```python
from build123d import *

# Parameters (mm, degrees)
SKETCH1_R          = 5.25
SKETCH1_R_2        = 10
SKETCH1_R_3        = 6.25
SKETCH1_R_4        = 4.25
BASE_FLANGE1_DEPTH = 4
FILLET1_R          = 10


# Sheet-metal steps are written as plain solids
with BuildPart() as part:
    # Sketch1 → Base-Flange1 (new body)
    with BuildSketch(Plane(origin=(0, 0, 0), x_dir=(1, 0, 0), z_dir=(0, 1, 0))):
        Polygon((70, -42.5), (-70, -42.5), (-70, 42.5), (-70, 72.5), (230, 72.5), (230, 42.5), (70, 42.5), align=None)
        with Locations(Location((-55, 57.5, 0), (0, 0, 270))):
            Circle(SKETCH1_R, mode=Mode.SUBTRACT)
        with Locations(Location((215, 57.5, 0), (0, 0, 270))):
            Circle(SKETCH1_R, mode=Mode.SUBTRACT)
        with Locations(Location((0, -17.5, 0), (0, 0, 270))):
            Circle(SKETCH1_R_2, mode=Mode.SUBTRACT)
        with Locations(Location((-45, -17.5, 0), (0, 0, 270))):
            Circle(SKETCH1_R_3, mode=Mode.SUBTRACT)
        with Locations(Location((45, -17.5, 0), (0, 0, 270))):
            Circle(SKETCH1_R_3, mode=Mode.SUBTRACT)
        with Locations(Location((-45, 12.5, 0), (0, 0, 270))):
            Circle(SKETCH1_R_4, mode=Mode.SUBTRACT)
        with Locations(Location((45, 12.5, 0), (0, 0, 270))):
            Circle(SKETCH1_R_4, mode=Mode.SUBTRACT)
    extrude(amount=-BASE_FLANGE1_DEPTH)

    # Fillet1
    fillet1_edges = [part.edges().sort_by_distance(p)[0] for p in [
        (-70, -2, -72.5),
        (230, -2, -72.5),
        (230, -2, -42.5),
        (70, -2, -42.5),
        (70, -2, 42.5),
        (-70, -2, 42.5),
    ]]
    fillet(fillet1_edges, radius=FILLET1_R)


solid = part.part
```
Source: CAD feature listing. Evaluate the final solid. Frame: model axes, mm. Give positions to 0.01 mm unless a question says otherwise; leave off trailing zeros. Write each loop counter-clockwise with the first axis right and the second up, starting at its lowest first coordinate (ties: lowest second). Pieces come first, ordered by that corner, then holes.
1. Section query B-B (z = 17.5). Return the cut outline in (x, y), then the cut area to 3 significant figures.
2. Section query D-D (z = -57.5). Return the cut outline in (x, y), then the cut area to 3 significant figures.
3. First-contact query: pin 1 (7 mm diameter, centred on x = 45, z = -12.5, fed in from -Y); pin 2 (2 mm diameter, centred on y = -1.5, z = -10, fed in from +X). Flat tips, straight axial feed; report the tip coordinate or a pass-through.
4. Pull-direction query (Z, two-part tool) for faces 1 (the face through (66.99, -2.03, 39.65)), 2 (the face through (-67.15, -2.03, -69.49)), 3 (the face through (51.2, -2, 16.7)); classes: +Z half, -Z half, draft (parallel to the pull), parting line (faces both ways), or undercut.
5. Section query C-C (x = 45). Return the cut outline in (y, z), then the cut area to 3 significant figures.
6. Material intervals for line 1 along X through (y, z) = (-0.95, 17.5); line 2 along X through (y, z) = (-2.05, -57.5); line 3 along X through (y, z) = (-2.8, 15.5), sorted ascending.
7. Section query A-A (x = 0). Return the cut outline in (y, z), then the cut area to 3 significant figures.
Output values:
1. outline: (-70, -4) - (-51.25, -4) - (-51.25, 0) - (-70, 0) - close; (-38.75, -4) - (-10, -4) - (-10, 0) - (-38.75, 0) - close; (10, -4) - (38.75, -4) - (38.75, 0) - (10, 0) - close; (51.25, -4) - (70, -4) - (70, 0) - (51.25, 0) - close
1. area: 380 mm2
2. outline: (-70, -4) - (-60.25, -4) - (-60.25, 0) - (-70, 0) - close; (-49.75, -4) - (209.75, -4) - (209.75, 0) - (-49.75, 0) - close; (220.25, -4) - (230, -4) - (230, 0) - (220.25, 0) - close
2. area: 1,120 mm2
3. pin 1: passes through
3. pin 2: stops at x = 70
4. face 1: +Z half
4. face 2: -Z half
4. face 3: undercut
5. outline: (-4, -72.5) - (0, -72.5) - (0, -16.75) - (-4, -16.75) - close; (-4, -8.25) - (0, -8.25) - (0, 11.25) - (-4, 11.25) - close; (-4, 23.75) - (0, 23.75) - (0, 42.5) - (-4, 42.5) - close
5. area: 376 mm2
6. line 1: x = -70 to -51.25, -38.75 to -10, 10 to 38.75, 51.25 to 70
6. line 2: x = -70 to -60.25, -49.75 to 209.75, 220.25 to 230
6. line 3: x = -70 to -50.92, -39.08 to -9.8, 9.8 to 39.08, 50.92 to 70
7. outline: (-4, -72.5) - (0, -72.5) - (0, 7.5) - (-4, 7.5) - close; (-4, 27.5) - (0, 27.5) - (0, 42.5) - (-4, 42.5) - close
7. area: 380 mm2
